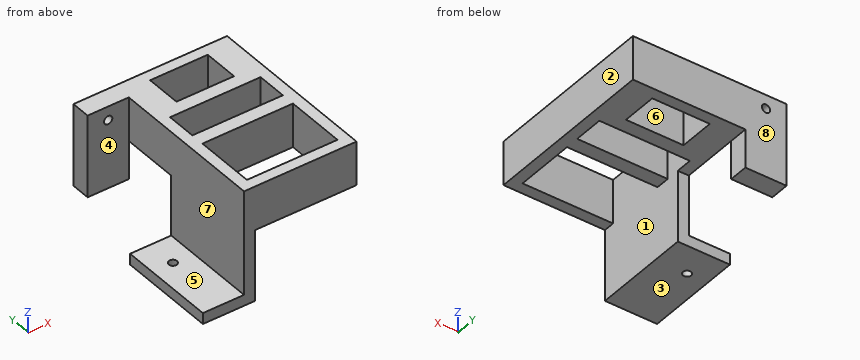
from build123d import *

# Parameters (mm, degrees)
CROQUIS1_W              = 41
CROQUIS1_H              = 64
CROQUIS1_W_2            = 33
CROQUIS1_H_2            = 22
CROQUIS1_H_3            = 11
CROQUIS1_W_3            = 21
CROQUIS1_H_4            = 13
SALIENTE_EXTRUIR1_DEPTH = 16
CROQUIS2_W              = 30
CROQUIS2_H              = 7
SALIENTE_EXTRUIR2_DEPTH = 15
SALIENTE_EXTRUIR3_DEPTH = 22
CROQUIS4_W              = 4
CROQUIS4_H              = 36
SALIENTE_EXTRUIR4_DEPTH = 19
CORTAR_EXTRUIR3_START   = -7
CROQUIS5_R              = 1.5
CORTAR_EXTRUIR3_DEPTH   = 7
CROQUIS7_R              = 1.5
CORTAR_EXTRUIR6_DEPTH   = 4


with BuildPart() as part:
    # Croquis1 → Saliente-Extruir1 (new body)
    with BuildSketch(Plane.XY):
        with Locations((-82.994239819, 12.027777778)):
            Rectangle(CROQUIS1_W, CROQUIS1_H)
        with Locations((-82.994239819, -4.972222222)):
            Rectangle(CROQUIS1_W_2, CROQUIS1_H_2, mode=Mode.SUBTRACT)
        with Locations((-82.994239819, 16.527777778)):
            Rectangle(CROQUIS1_W_2, CROQUIS1_H_3, mode=Mode.SUBTRACT)
        with Locations((-82.994239819, 33.527777778)):
            Rectangle(CROQUIS1_W_3, CROQUIS1_H_4, mode=Mode.SUBTRACT)
    extrude(amount=SALIENTE_EXTRUIR1_DEPTH)

    # Croquis2 → Saliente-Extruir2 (add)
    with BuildSketch(Plane.ZY.offset(103.494239819)):
        with Locations((1, 40.527777778)):
            Rectangle(CROQUIS2_W, CROQUIS2_H)
    extrude(amount=SALIENTE_EXTRUIR2_DEPTH)

    # Croquis3 → Saliente-Extruir3 (add)
    with BuildSketch(Plane(origin=(0, 0, 0), x_dir=(-1, 0, 0), z_dir=(0, 0, -1))):
        Polygon((103.494239819, -19.972222222), (99.494239819, -19.972222222), (99.494239819, 6.027777778), (99.494239819, 16.027777778), (103.494239819, 16.027777778), (103.494239819, 6.027777778), align=None)
    extrude(amount=SALIENTE_EXTRUIR3_DEPTH)

    # Croquis4 → Saliente-Extruir4 (add)
    with BuildSketch(Plane(origin=(-99.494239819, 0, 0), x_dir=(0, 0, -1), z_dir=(1, 0, 0))):
        with Locations((24, -1.972222222)):
            Rectangle(CROQUIS4_W, CROQUIS4_H)
    extrude(amount=-SALIENTE_EXTRUIR4_DEPTH)

    # Croquis5 → Cortar-Extruir3 (cut)
    with BuildSketch(Plane(origin=(0, 44.027777778, 0), x_dir=(1, 0, 0), z_dir=(0, 1, 0)).offset(CORTAR_EXTRUIR3_START)):
        with Locations((-110.994239819, -11)):
            Circle(CROQUIS5_R)
    extrude(amount=CORTAR_EXTRUIR3_DEPTH, mode=Mode.SUBTRACT)

    # Croquis7 → Cortar-Extruir6 (cut)
    with BuildSketch(Plane.XY.offset(-22)):
        with Locations((-110.994239819, 5.027777778)):
            Circle(CROQUIS7_R)
    extrude(amount=-CORTAR_EXTRUIR6_DEPTH, mode=Mode.SUBTRACT)


solid = part.part
Source: CAD feature listing. Evaluate the final solid. Frame: model axes, mm. Face numbers are marked on the shaded views. A direction names the side the tool comes from. Give positions to 0.01 mm unless a question says otherwise; leave off trailing zeros. Write each loop counter-clockwise with the first axis right and the second up, starting at its lowest first coordinate (ties: lowest second). Pieces come first, ordered by that corner, then holes. Notation, with made-up numbers: M 0.5,79.25 L 57.5,79.25 A16 cw 57.5,91.25 Z; hole C 16.5,74 d1. An arc over 180 degrees is marked long. Answer as a JSON object with one key per item and string values.
Q1. Mould query, pull axis X, two halves, no side actions, for the marked faces 1, 2 and 3. Classes: +X half, -X half, draft (parallel to the pull), parting line (faces both ways), or undercut.
Geometry check:
{"face 1": "undercut", "face 2": "+X half", "face 3": "draft"}
Q2. Cut plane B-B, the plane z = -2. Return the cut outline in (x, y).
Geometry check:
{"outline": "M -118.49,37.03 L -103.49,37.03 L -103.49,44.03 L -118.49,44.03 Z; M -103.49,-19.97 L -99.49,-19.97 L -99.49,16.03 L -103.49,16.03 Z"}
Q3. Cut plane A-A, the plane y = -11.5. Return the cut outline in (x, z).
Geometry check:
{"outline": "M -118.49,-26 L -99.49,-26 L -99.49,16 L -103.49,16 L -103.49,-22 L -118.49,-22 Z; M -66.49,0 L -62.49,0 L -62.49,16 L -66.49,16 Z"}
Q4. Contact query for flat-ended pins moving along their axis: P1, Ø7.5, axis at x = -108, y = 41, coming from the -Z side; P2, Ø10, axis at x = -78.5, y = 1.5, coming from the -Z side; P3, Ø4.5, axis at x = -109.5, y = -8.5, coming from the +Z side. Output: stop coordinate, or through.
Geometry check:
{"P1": "stops at z = -14", "P2": "stops at z = 0", "P3": "stops at z = -22"}
Q5. Access query for the marked faces 4, 5, 6, 7 and 8. Directions: +Z, -Z, +X, -X, +Y, -Y. A direction counts if a zero-diameter tool reaches every point of the face in a straight line with its end or side. Return the directions, or none.
Geometry check:
{"face 4": "+Z, -Z, -X, -Y", "face 5": "+Z, -X, +Y, -Y", "face 6": "+Z, -Z", "face 7": "+Z, -X, -Y", "face 8": "+Z, -Z, +X, -X, +Y"}
Q6. Cut plane D-D, the plane z = 11. Return the cut outline in (x, y), then the cut area to 3 significant figures.
Geometry check:
{"outline": "M -118.49,37.03 L -112.49,37.03 L -112.49,44.03 L -118.49,44.03 Z; M -109.49,37.03 L -103.49,37.03 L -103.49,-19.97 L -62.49,-19.97 L -62.49,44.03 L -109.49,44.03 Z; hole M -99.49,-15.97 L -66.49,-15.97 L -66.49,6.03 L -99.49,6.03 Z; hole M -99.49,11.03 L -66.49,11.03 L -66.49,22.03 L -99.49,22.03 Z; hole M -93.49,27.03 L -72.49,27.03 L -72.49,40.03 L -93.49,40.03 Z", "area": "1,350 mm^2"}
Q7. Cut plane C-C, the plane x = -105. Return the cut outline in (y, z), then the cut area to 3 significant figures.
Geometry check:
{"outline": "M -19.97,-26 L 16.03,-26 L 16.03,-22 L -19.97,-22 Z; M 37.03,-14 L 44.03,-14 L 44.03,16 L 37.03,16 Z", "area": "354 mm^2"}
Q8. Ray query, line 1 along X through (y, z) = (39, 11); line 2 along Y through (x, z) = (-87, 6.5); line 3 along Y through (x, z) = (-71, 4.5). Return the intervals inside material, ascending.
Geometry check:
{"line 1": "x = -118.49 to -112.49, -109.49 to -93.49, -72.49 to -62.49", "line 2": "y = -19.97 to -15.97, 6.03 to 11.03, 22.03 to 27.03, 40.03 to 44.03", "line 3": "y = -19.97 to -15.97, 6.03 to 11.03, 22.03 to 44.03"}
